Check sheet for the modelled part. Datum: model origin and axes. Units: mm. A direction names the side the tool comes from. Give positions to 0.01 mm unless a question says otherwise; leave off trailing zeros. Order: outer loops, then holes, each group sorted by start corner. A loop starts at its lowest first (then second) coordinate and runs counter-clockwise, first axis right, second up.
```python
from build123d import *

# Parameters (mm, degrees)
BOSS_EXTRUDE1_DEPTH      = 60
SKETCH2_R                = 8.5
CUT_EXTRUDE1_DEPTH       = 60
BOSS_EXTRUDE2_DEPTH      = 15
SKETCH3_R                = 16
SKETCH3_R_2              = 11
BOSS_EXTRUDE3_DEPTH      = 20
BOSS_EXTRUDE3_DEPTH_BACK = 20
CUT_EXTRUDE2_DEPTH       = 57


with BuildPart() as part:
    # Sketch1 → Boss-Extrude1 (new body)
    with BuildSketch(Plane(origin=(0, 0, 0), x_dir=(0, 0, -1), z_dir=(1, 0, 0))):
        Polygon((-31.570634591, -10.443354749), (-31.570634591, -28.443354749), (23.429365409, -28.443354749), (23.429365409, -40.443354749), (43.429365409, -40.443354749), (43.429365409, -10.443354749), align=None)
    extrude(amount=BOSS_EXTRUDE1_DEPTH)

    # Sketch2 → Cut-Extrude1 (cut)
    with BuildSketch(Plane(origin=(0, -10.443354749, 0), x_dir=(1, 0, 0), z_dir=(0, 1, 0))):
        with Locations(Location((35, -19.570634591, 0), (0, 0, 270))):
            Circle(SKETCH2_R)
        with Locations(Location((35, 5.429365409, 0), (0, 0, 270))):
            Circle(SKETCH2_R)
    extrude(amount=-CUT_EXTRUDE1_DEPTH, mode=Mode.SUBTRACT)

    # 3DSketch1 → Boss-Extrude2 (add)
    with BuildSketch(Plane(origin=(0, -10.443354749, 31.570634591), x_dir=(0, 0.28727544621498696, -0.9578480140408394), z_dir=(1, 0, 0))):
        Polygon((0, 0), (71.838601053, -21.545658466), (155.320085422, 0), (146.20131027, 30.673244689), (102.486579182, 11.022753171), align=None)
    extrude(amount=BOSS_EXTRUDE2_DEPTH)

    # Sketch3 → Boss-Extrude3 (add, two sides)
    with BuildSketch(Plane(origin=(15, 0, 0), x_dir=(0, 0, -1), z_dir=(1, 0, 0))) as boss_extrude3_sk:
        with Locations((108.429365409, 47.556645251)):
            Circle(SKETCH3_R)
        with Locations((108.429365409, 47.556645251)):
            Circle(SKETCH3_R_2, mode=Mode.SUBTRACT)
    extrude(amount=BOSS_EXTRUDE3_DEPTH)
    extrude(boss_extrude3_sk.sketch, amount=-BOSS_EXTRUDE3_DEPTH_BACK)

    # Sketch4 → Cut-Extrude2 (cut)
    with BuildSketch(Plane(origin=(15, 0, 0), x_dir=(0, 0, -1), z_dir=(1, 0, 0))):
        with BuildLine():
            Line((114.460827221, 38.357652457), (102.397903597, 56.755638044))
            ThreePointArc((102.397903597, 56.755638044), (99.230372615, 41.525183439), (114.460827221, 38.357652457))
        make_face()
    extrude(amount=-CUT_EXTRUDE2_DEPTH, mode=Mode.SUBTRACT)


solid = part.part
```
(1) Cross-section at C-C on x = 54. Enter the section's corners in (y, z), then the cut area to 3 significant figures.
Response values:
outline: (-40.44, -43.43) - (-10.44, -43.43) - (-10.44, 31.57) - (-28.44, 31.57) - (-28.44, -23.43) - (-40.44, -23.43) - close
area: 1,590 mm2
(2) Cross-section at D-D on z = -46.5. Enter the section's corners in (x, y).
Response values:
outline: (0, -8.59) - (15, -8.59) - (15, 22.43) - (0, 22.43) - close
(3) Release check for a two-part mould opening along X. For faces 6 (the face through (7.4, 44.05, -80.16)), 7 (the face through (35, 44.2, -97.5)), 8 (the face through (27.459, -19.317, 23.493)) record: released by +X, released by -X, zero draft, split by the parting line, or undercut.
Response values:
face 6: zero draft
face 7: released by +X
face 8: undercut
(4) Material ranges on L1, parallel to Y at x = 54, z = -42.5; L2, parallel to Y at x = 20, z = 21; L3, parallel to Y at x = 34.5, z = -107, recorded low to high.
Response values:
L1: y = -40.44 to -10.44
L2: y = -28.44 to -10.44
L3: y = 31.62 to 36.65, 58.46 to 63.49
(5) Set-up check for faces 1 (the face through (7.395, 9.837, -16.594)), 2 (the face through (30, -26, -43.429)), 3 (the face through (30, -19, 31.571)), 4 (the face through (30, -34, -23.429)), 5 (the face through (37, -10.443, -15)): record each of +Z, -Z, +X, -X, +Y, -Y from which the full face is reachable in a straight line by a thin tool's end or side.
Response values:
face 1: +Z, +X, -X, +Y
face 2: -Z, +X, -X, -Y
face 3: +Z, +X, -X, +Y, -Y
face 4: +Z, +X, -X, -Y
face 5: +Z, -Z, +X, +Y
(6) Cross-section at A-A on y = 49.5. Enter the section's corners in (x, z).
Response values:
outline: (-5, -124.31) - (35, -124.31) - (35, -119.26) - (-5, -119.26) - close; (-5, -97.6) - (35, -97.6) - (35, -92.55) - (15, -92.55) - (15, -86.45) - (0, -86.45) - (0, -92.55) - (-5, -92.55) - close
(7) Gauge pin test, flat ends, axial feed: pin 1 Ø1.5 at (y, z) = (27, -51.5) entering from -X; pin 2 Ø9 at (x, y) = (42, -20.5) entering from -Z; pin 3 Ø6 at (x, y) = (12.5, 5.5) entering from +Z; pin 4 Ø6 at (x, y) = (18, -33) entering from +Z. Record the tip position at first contact, or that the pin passes through.
Response values:
pin 1: passes through
pin 2: stops at z = -43.43
pin 3: stops at z = 0.83
pin 4: stops at z = -23.43
(8) Cross-section at B-B on x = 30.5. Enter the section's corners in (y, z).
Response values:
outline: (-40.44, -43.43) - (-10.44, -43.43) - (-10.44, -12.64) - (-28.44, -12.64) - (-28.44, -23.43) - (-40.44, -23.43) - close; (-28.44, 1.78) - (-10.44, 1.78) - (-10.44, 12.36) - (-28.44, 12.36) - close; (-28.44, 26.78) - (-10.44, 26.78) - (-10.44, 31.57) - (-28.44, 31.57) - close; circle Ø32 at (47.56, -108.43); hole circle Ø22 at (47.56, -108.43)
